from build123d import *

# Parameters (mm, degrees)
F1_DEPTH = 5
F3_R     = 1.5
F4_DEPTH = 4
F2_R     = 1.5
F5_DEPTH = 4


with BuildPart() as f1:
    # F0 (on Right) → F1 (new body)
    with BuildSketch(Plane.YZ):
        Polygon((9.9999599028, -0.028318582), (0, 0), (0, -5), (9.9999599028, -4.971681418), (14.6977243388, -3.2596623456), (12.8266741155, 0.9765131251), align=None)
        with BuildLine():
            Line((0, -5), (0, 0))
            ThreePointArc((0, 0), (-2.5070896982, -2.5), (0, -5))
        make_face()
    extrude(amount=F1_DEPTH)

    # F3 (on face) → F4 (join)
    with BuildSketch(Plane.YZ.offset(5)):
        with Locations((-0.0070796739, -2.5)):
            Circle(F3_R)
    extrude(amount=F4_DEPTH)

    # F2 (on face) → F5 (join)
    with BuildSketch(Plane(origin=(0, 11.0937619601, 4.8999353157), x_dir=(-1, 0, 0), z_dir=(0, 0.9147463248, 0.4040286639))):
        with Locations((-2.5, -6.6045741447)):
            Circle(F2_R)
    extrude(amount=F5_DEPTH)


solid = f1.part
Design review of the part built by this model. Coordinates are the model's own, in mm. A direction names the side the tool comes from. Give positions to 0.01 mm unless a question says otherwise; leave off trailing zeros. Loops run counter-clockwise (first coordinate to the right, second up) from the corner with the lowest first, then second, coordinate; pieces in that order, holes last. Notation, with made-up numbers: (55.5, -4.75) -> (93.5, -4.75) arc R27 ccw to (93.5, 30.25) -> close; hole circle Ø5 at (25, -33). An arc over 180 degrees is marked (long way). One line per question, with ' | ' between items. Start each with the question number.
(1) We need section C-C (y = 6.25). State the section outline as (x, z) points, and give its area (3 significant figures).
(2) We need section D-D (x = 7.5). State the section outline as (y, z) points, and give its area (3 significant figures).
(3) We need section B-B (z = -3). State the section outline as (x, y) points, and give its area (3 significant figures).
(4) For faces 4 (the face through (9, 0, -2)), 5 (the face through (1.909, 14.399, -2.583)), 6 (the face through (7, 0, -1)), list the 3-axis set-ups (+Z, -Z, +X, -X, +Y, -Y) from which the entire face can be reached by the end or side of a thin tool; tool diameter is ignored.
(5) We need section A-A (x = 3). State the section outline as (y, z) points, and give its area (3 significant figures).
(6) Draft analysis for pull direction Y (two halves, no side actions). For faces 1 (the face through (2.521, 17.413, 0.494)), 2 (the face through (0, 6, -3)), 3 (the face through (1.114, 15.798, -0.87)), state which applies: +Y half, -Y half, draft (parallel to the pull), parting line (faces both ways), or undercut.
(7) Insertion check: P1, Ø1.5, axis at x = 2.5, y = 4.5, coming from the -Z side; P2, Ø1.8, axis at y = 7.5, z = -0.5, coming from the +X side; P3, Ø1, axis at x = 2.5, z = -0.5, coming from the -Y side. Each pin has a flat end and moves straight along its axis. Give the tip position at first contact, or say it passes through.
(8) For line 1 (X direction, y = 0.5, z = -0.5); line 2 (Z direction, x = 4.75, y = 2.5); line 3 (Y direction, x = 6.5, z = -3.5), list the stretches that pass through material, from the lowest coordinate up.
The answers:
1) outline: (0, -4.98) -> (5, -4.98) -> (5, -0.02) -> (0, -0.02) -> close | area: 24.8 mm^2
2) outline: circle Ø3 at (-0.01, -2.5) | area: 7.07 mm^2
3) outline: (0, -2.46) -> (5, -2.46) -> (5, -1.42) -> (9, -1.42) -> (9, 1.41) -> (5, 1.41) -> (5, 14.58) -> (0, 14.58) -> close | area: 96.5 mm^2
4) face 4: +Z, -Z, +X, +Y, -Y | face 5: none | face 6: +X
5) outline: (0, -5) -> (10, -4.97) -> (14.7, -3.26) -> (14.33, -2.44) -> (17.99, -0.82) -> (16.85, 1.77) -> (13.19, 0.15) -> (12.83, 0.98) -> (10, -0.03) -> (0, 0) arc R2.5 ccw (long way) to start | area: 89.4 mm^2
6) face 1: +Y half | face 2: draft | face 3: undercut
7) P1: stops at z = -4.99 | P2: stops at x = 5 | P3: stops at y = -2.01
8) line 1: x = 0 to 5 | line 2: z = -4.99 to -0.01 | line 3: y = -1.13 to 1.11
